Work out the finished part from the listing and answer in its coordinate system (mm). Face numbers are marked on the shaded views. A direction names the side the tool comes from. Round coordinates to 2 decimals unless told otherwise and drop trailing zeros. Write each loop counter-clockwise with the first axis right and the second up, starting at its lowest first coordinate (ties: lowest second). Pieces come first, ordered by that corner, then holes. Notation, with made-up numbers: (74.5, 1.5) - (125.5, 1.5) arc R25 ccw to (125.5, 32.5) - close; hole circle Ø1 at (53, 88). An arc over 180 degrees is marked (long way). Answer as a JSON object with one key per item and string values.
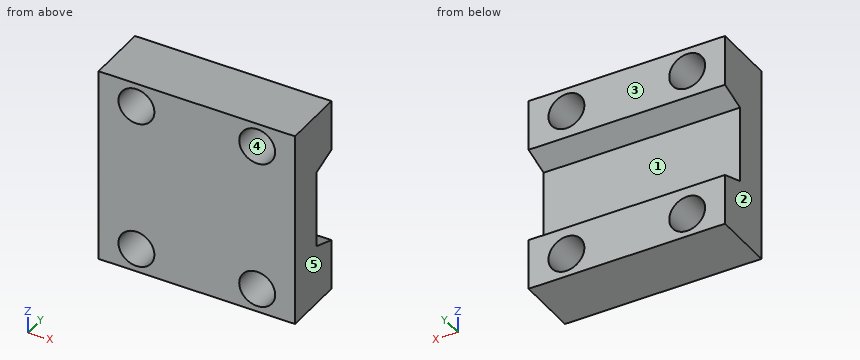
```python
from build123d import *

# Parameters (mm, degrees)
SKETCH1_W                            = 38.29
SKETCH1_H                            = 38.3
BOSS_EXTRUDE1_DEPTH                  = 12.12
CUT_EXTRUDE1_DEPTH                   = 45.494280531
M8X1_0_TAPPED_HOLE2_D                = 7
MIRROR1_AT_THE_SECOND_PLANE_COPY_1_D = 7


with BuildPart() as part:
    # Sketch1 → Boss-Extrude1 (new body)
    with BuildSketch(Plane(origin=(0, 0, 0), x_dir=(1, 0, 0), z_dir=(0, 1, 0))):
        Rectangle(SKETCH1_W, SKETCH1_H)
    extrude(amount=BOSS_EXTRUDE1_DEPTH)

    # Sketch2 → Cut-Extrude1 (cut, through all)
    with BuildSketch(Plane(origin=(19.145, 0, 0), x_dir=(0, 0, -1), z_dir=(1, 0, 0))):
        with BuildLine():
            Line((8.348193896, 12.12), (-7.620525527, 12.12))
            ThreePointArc((-7.620525527, 12.12), (-7.350184436, 9.500113986), (-6.243729663, 7.11))
            Line((-6.243729663, 7.11), (6.971398032, 7.11))
            ThreePointArc((6.971398032, 7.11), (8.007802748, 9.259969363), (8.363834185, 11.62))
            ThreePointArc((8.363834185, 11.62), (8.359923156, 11.870122279), (8.348193896, 12.12))
        make_face()
        with BuildLine():
            Line((-7.620525527, 12.12), (-9.216421688, 12.12))
            Line((-9.216421688, 12.12), (-7.5, 7.11))
            Line((-7.5, 7.11), (-6.243729663, 7.11))
            ThreePointArc((-6.243729663, 7.11), (-7.350184436, 9.500113986), (-7.620525527, 12.12))
        make_face()
        with BuildLine():
            Line((9.216421688, 12.12), (8.348193896, 12.12))
            ThreePointArc((8.348193896, 12.12), (8.359923156, 11.870122279), (8.363834185, 11.62))
            ThreePointArc((8.363834185, 11.62), (8.007802748, 9.259969363), (6.971398032, 7.11))
            Line((6.971398032, 7.11), (7.5, 7.11))
            Line((7.5, 7.11), (9.216421688, 12.12))
        make_face()
    extrude(amount=-CUT_EXTRUDE1_DEPTH, mode=Mode.SUBTRACT)

    # M8x1.0 Tapped Hole2 (through all)
    with Locations(Plane(origin=(0, 12.12, 0), x_dir=(1, 0, 0), z_dir=(0, 1, 0))):
        with Locations((-11.77, 14.55), (11.77, 14.55), (-11.77, -14.55), (11.77, -14.55)):
            m8x1_0_tapped_hole2 = Hole(M8X1_0_TAPPED_HOLE2_D / 2)

    # Mirror1: M8x1.0 Tapped Hole2 across plane
    add(m8x1_0_tapped_hole2.mirror(Plane.XY), mode=Mode.SUBTRACT)

    # Mirror1 at the second plane: M8x1.0 Tapped Hole2 across plane
    add(m8x1_0_tapped_hole2.mirror(Plane(origin=(0, 0, 0), x_dir=(0, 0, 1), z_dir=(1, 0, 0))), mode=Mode.SUBTRACT)

    # Mirror1 at the second plane copy 1 (through all)
    with Locations(Plane(origin=(0, 12.12, 0), x_dir=(-1, 0, 0), z_dir=(0, 1, 0))):
        with Locations((-11.77, 14.55), (11.77, 14.55), (-11.77, -14.55), (11.77, -14.55)):
            Hole(MIRROR1_AT_THE_SECOND_PLANE_COPY_1_D / 2)


solid = part.part
```
Item 1: A cutting plane is placed at C-C (z = 14.55). Write down the section's boundary in (x, y) (3 decimals), and give its area (3 significant figures).
Results found:
{"outline": "(-19.145, 0) - (-15.27, 0) - (-15.27, 12.12) - (-19.145, 12.12) - close; (-8.27, 0) - (8.27, 0) - (8.27, 12.12) - (-8.27, 12.12) - close; (15.27, 0) - (19.145, 0) - (19.145, 12.12) - (15.27, 12.12) - close", "area": "294 mm²"}
Item 2: Determine the mould class of the marked faces 3, 4 and 5 for opening direction X: pulls with the +X half, pulls with the -X half, needs draft (parallel to the pull), parting line crosses it, or undercut.
Results found:
{"face 3": "needs draft", "face 4": "undercut", "face 5": "pulls with the +X half"}
Item 3: Each of these flat-tipped pins is pushed along its axis until it touches: P1, Ø4.5, axis at x = -9.5, z = -0.5, coming from the +Y side; P2, Ø6.5, axis at x = -11.77, z = -14.55, coming from the -Y side. Where does it stop, or does it pass through?
Results found:
{"P1": "y = 7.11", "P2": "through"}
Item 4: A cutting plane is placed at A-A (x = -11.77). Write down the section's boundary in (y, z), and give its area (3 significant figures).
Results found:
{"outline": "(0, -19.15) - (12.12, -19.15) - (12.12, -18.05) - (0, -18.05) - close; (0, -11.05) - (12.12, -11.05) - (12.12, -9.22) - (7.11, -7.5) - (7.11, 7.5) - (12.12, 9.22) - (12.12, 11.05) - (0, 11.05) - close; (0, 18.05) - (12.12, 18.05) - (12.12, 19.15) - (0, 19.15) - close", "area": "211 mm²"}
Item 5: A cutting plane is placed at D-D (x = -4). Write down the section's boundary in (y, z), and give its area (3 significant figures).
Results found:
{"outline": "(0, -19.15) - (12.12, -19.15) - (12.12, -9.22) - (7.11, -7.5) - (7.11, 7.5) - (12.12, 9.22) - (12.12, 19.15) - (0, 19.15) - close", "area": "380 mm²"}
Item 6: A cutting plane is placed at B-B (y = 2). Write down the section's boundary in (x, z) (3 decimals), and give its area (3 significant figures).
Results found:
{"outline": "(-19.145, -19.15) - (19.145, -19.15) - (19.145, 19.15) - (-19.145, 19.15) - close; hole circle Ø7 at (-11.77, -14.55); hole circle Ø7 at (-11.77, 14.55); hole circle Ø7 at (11.77, -14.55); hole circle Ø7 at (11.77, 14.55)", "area": "1,310 mm²"}
Item 7: For the marked faces 1 and 2, determine the directions among +Z, -Z, +X, -X, +Y, -Y from which every point of the face is accessible in a straight line to the end or side of a thin tool.
Results found:
{"face 1": "+X, -X, +Y", "face 2": "+Z, -Z, -X, +Y, -Y"}
Item 8: Consider line 1 along Z through (x, y) = (11.77, 3); line 2 along Z through (x, y) = (-11.77, 9.25); line 3 along X through (y, z) = (8.25, 13) (3 decimals). Determine where each line is inside the solid, lowest interval first.
Results found:
{"line 1": "-19.15 to -18.05, -11.05 to 11.05, 18.05 to 19.15", "line 2": "-19.15 to -18.05, -11.05 to -8.23, 8.23 to 11.05, 18.05 to 19.15", "line 3": "-19.145 to -14.908, -8.632 to 8.632, 14.908 to 19.145"}
